```python
from build123d import *

# Parameters (mm, degrees)
ESQUISSE1_R             = 7.48734248
ESQUISSE1_R_2           = 2.5
BOSS_EXTRU_1_DEPTH      = 5
ESQUISSE2_R             = 1.2295
ENL_V_MAT_EXTRU_1_DEPTH = 5
CONG_2_R                = 10
CONG_3_R                = 10
ESQUISSE3_R             = 11.25
ENL_V_MAT_EXTRU_2_DEPTH = 10
CHANFREIN1_SIZE         = 5


with BuildPart() as part:
    # Esquisse1 → Boss.-Extru.1 (new body)
    with BuildSketch(Plane.XY):
        with BuildLine():
            Line((-33.258331918, 42.564920159), (33.258331918, 42.564920159))
            ThreePointArc((33.258331918, 42.564920159), (42.517839876, 33.305412201), (33.258331918, 24.045904244))
            Line((33.258331918, 24.045904244), (21, 0))
            Line((21, 0), (21, -21))
            Line((21, -21), (-21, -21))
            Line((-21, -21), (-21, 0))
            Line((-21, 0), (-33.258331918, 24.045904244))
            ThreePointArc((-33.258331918, 24.045904244), (-42.517839876, 33.305412201), (-33.258331918, 42.564920159))
        make_face()
        Circle(ESQUISSE1_R, mode=Mode.SUBTRACT)
        with Locations((-33.258331918, 33.306233754)):
            Circle(ESQUISSE1_R_2, mode=Mode.SUBTRACT)
        with Locations(Location((33.258331918, 33.306233754, 0), (0, 0, 180))):
            Circle(ESQUISSE1_R_2, mode=Mode.SUBTRACT)
        with Locations((-15, 33.108389008)):
            Circle(ESQUISSE1_R_2, mode=Mode.SUBTRACT)
        with Locations(Location((15, 33.108389008, 0), (0, 0, 180))):
            Circle(ESQUISSE1_R_2, mode=Mode.SUBTRACT)
    extrude(amount=BOSS_EXTRU_1_DEPTH)

    # Esquisse2 → Enlèv. mat.-Extru.1 (cut)
    with BuildSketch(Plane.XY.offset(5)):
        with Locations((-15.5, 15.5)):
            Circle(ESQUISSE2_R)
        with Locations((15.5, 15.5)):
            Circle(ESQUISSE2_R)
        with Locations((-15.5, -15.5)):
            Circle(ESQUISSE2_R)
        with Locations((15.5, -15.5)):
            Circle(ESQUISSE2_R)
    extrude(amount=-ENL_V_MAT_EXTRU_1_DEPTH, mode=Mode.SUBTRACT)

    # Congé2
    cong_2_edges = [part.edges().sort_by_distance(p)[0] for p in [
        (-21, 0, 2.5),
        (21, 0, 2.5),
    ]]
    fillet(cong_2_edges, radius=CONG_2_R)

    # Congé3
    cong_3_edges = [part.edges().sort_by_distance(p)[0] for p in [
        (-33.258331918, 24.045904244, 2.5),
        (33.258331918, 24.045904244, 2.5),
    ]]
    fillet(cong_3_edges, radius=CONG_3_R)

    # Esquisse3 → Enlèv. mat.-Extru.2 (cut)
    with BuildSketch(Plane.XY.offset(5)):
        Circle(ESQUISSE3_R)
    extrude(amount=-ENL_V_MAT_EXTRU_2_DEPTH, mode=Mode.SUBTRACT)

    # Chanfrein1
    chanfrein1_edges = [part.edges().sort_by_distance(p)[0] for p in [
        (21, -21, 2.5),
        (-21, -21, 2.5),
    ]]
    chamfer(chanfrein1_edges, length=CHANFREIN1_SIZE)


solid = part.part
```
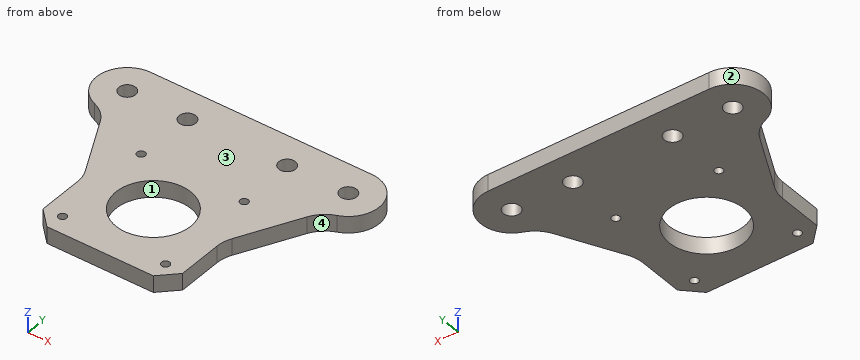
CAD build for the part. Positions are in the model's coordinates, mm. Face numbers are marked on the shaded views. Round coordinates to 2 decimals unless told otherwise and drop trailing zeros. Loops run counter-clockwise (first coordinate to the right, second up) from the corner with the lowest first, then second, coordinate; pieces in that order, holes last. Notation, with made-up numbers: M 29.25,-12 L 65.25,-12 A19 cw 65.25,21 Z; hole C -28.5,80 d4. An arc over 180 degrees is marked long. Return JSON: item names as keys, results as strings. Group by question number.
(1) Saw through at C-C, the plane z = 2.95. Give the number of separate pieces and of enclosed holes in the cut face, and give its area (3 significant figures).
(2) Saw through at A-A, the plane x = 0. List the corners of the cut face in (y, z), and give its area (3 significant figures).
(3) Saw through at B-B, the plane y = 9. List the corners of the cut face in (x, z), and give its area (3 significant figures).
(4) Drop flat-ended pins along their axis: P1, Ø1.5, axis at y = -10.5, z = 2.5, coming from the -X side; P2, Ø4, axis at x = -33.26, y = 33.31, coming from the -Z side; P3, Ø2.5, axis at y = -8.5, z = 1.5, coming from the +X side. Give the stop position or say it passes through.
(5) Wall check: probe 1 along Y at (x, z) = (0, 2.9); probe 2 along X at (y, z) = (16, 1.5); probe 3 along Y at (x, z) = (15, 3.35). Give the ranges that are in metal, low to high. Write a range as [from, to].
(6) Saw through at D-D, the plane y = 23. List the corners of the cut face in (x, z).
(7) Mould opens along X. For the marked faces 1, 2, 3 and 4 say: +X half, -X half, draft (parallel to the pull), parting line (faces both ways), or undercut.
Answer list:
{
 "1": {"separate pieces": "1", "enclosed holes": "9", "area": "3,170 mm2"},
 "2": {"outline": "M -21,0 L -11.25,0 L -11.25,5 L -21,5 Z; M 11.25,0 L 42.56,0 L 42.56,5 L 11.25,5 Z", "area": "205 mm2"},
 "3": {"outline": "M -25.59,0 L -6.75,0 L -6.75,5 L -25.59,5 Z; M 6.75,0 L 25.59,0 L 25.59,5 L 6.75,5 Z", "area": "188 mm2"},
 "4": {"P1": "x = -21", "P2": "through", "P3": "x = 21"},
 "5": {"probe 1": "[-21, -11.25], [11.25, 42.56]", "probe 2": "[-29.16, -16.62], [-14.38, 14.38], [16.62, 29.16]", "probe 3": "[-21, -16.62], [-14.38, 14.38], [16.62, 30.61], [35.61, 42.56]"},
 "6": {"outline": "M -33.67,0 L 33.67,0 L 33.67,5 L -33.67,5 Z"},
 "7": {"face 1": "undercut", "face 2": "-X half", "face 3": "draft", "face 4": "+X half"}
}
